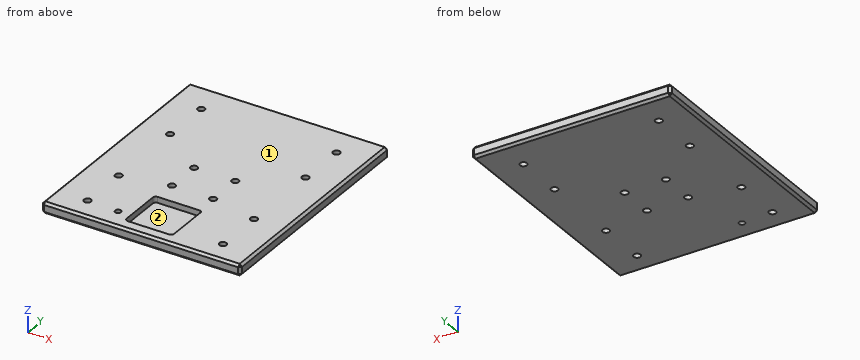
```python
from build123d import *

# Parameters (mm, degrees)
SKETCH1_W           = 107.95
SKETCH1_H           = 127
BOSS_EXTRUDE1_DEPTH = 6.223
CHAMFER1_SIZE       = 1.27
SKETCH2_R           = 1.905
CUT_EXTRUDE1_DEPTH  = 7.223
SKETCH3_R           = 1.905
CUT_EXTRUDE2_DEPTH  = 7.223
SKETCH4_W           = 25.781
SKETCH4_H           = 25.781
CUT_EXTRUDE3_DEPTH  = 3.175
FILLET1_R           = 1.5875
SKETCH5_R           = 1.5875
CUT_EXTRUDE4_DEPTH  = 7.223


with BuildPart() as part:
    # Sketch1 → Boss-Extrude1 (new body)
    with BuildSketch(Plane.XY):
        Rectangle(SKETCH1_W, SKETCH1_H)
    extrude(amount=BOSS_EXTRUDE1_DEPTH)

    # Chamfer1
    chamfer1_edges = [part.edges().sort_by_distance(p)[0] for p in [
        (-53.975, 0, 6.223),
        (0, -63.5, 6.223),
        (53.975, 0, 6.223),
        (0, -63.5, 0),
        (-53.975, 0, 0),
        (0, 63.5, 0),
        (53.975, 0, 0),
        (0, 63.5, 6.223),
        (53.975, -63.5, 3.1115),
        (-53.975, -63.5, 3.1115),
        (-53.975, 63.5, 3.1115),
        (53.975, 63.5, 3.1115),
    ]]
    chamfer(chamfer1_edges, length=CHAMFER1_SIZE)

    # Sketch2 → Cut-Extrude1 (cut, through all)
    with BuildSketch(Plane.XY.offset(6.223)):
        with Locations((-36.703, 46.228)):
            Circle(SKETCH2_R)
        with Locations((-36.703, -51.308)):
            Circle(SKETCH2_R)
        with Locations((36.703, -51.308)):
            Circle(SKETCH2_R)
        with Locations((36.703, 46.228)):
            Circle(SKETCH2_R)
        with Locations((-36.703, 19.558)):
            Circle(SKETCH2_R)
        with Locations((-36.703, -24.638)):
            Circle(SKETCH2_R)
        with Locations((36.703, 19.558)):
            Circle(SKETCH2_R)
        with Locations((36.703, -24.638)):
            Circle(SKETCH2_R)
    extrude(amount=-CUT_EXTRUDE1_DEPTH, mode=Mode.SUBTRACT)

    # Sketch3 → Cut-Extrude2 (cut, through all)
    with BuildSketch(Plane.XY.offset(6.223)):
        with Locations((-11.176, -0.254)):
            Circle(SKETCH3_R)
        with Locations((11.176, -0.254)):
            Circle(SKETCH3_R)
        with Locations((11.176, -19.304)):
            Circle(SKETCH3_R)
        with Locations((-11.176, -19.304)):
            Circle(SKETCH3_R)
    extrude(amount=-CUT_EXTRUDE2_DEPTH, mode=Mode.SUBTRACT)

    # Sketch4 → Cut-Extrude3 (cut)
    with BuildSketch(Plane.XY.offset(6.223)):
        with Locations((0, -44.2595)):
            Rectangle(SKETCH4_W, SKETCH4_H)
    extrude(amount=-CUT_EXTRUDE3_DEPTH, mode=Mode.SUBTRACT)

    # Fillet1
    fillet1_edges = [part.edges().sort_by_distance(p)[0] for p in [
        (12.8905, -31.369, 4.6355),
        (12.8905, -57.15, 4.6355),
        (-12.8905, -57.15, 4.6355),
        (-12.8905, -31.369, 4.6355),
    ]]
    fillet(fillet1_edges, radius=FILLET1_R)

    # Sketch5 → Cut-Extrude4 (cut, through all)
    with BuildSketch(Plane.XY.offset(6.223)):
        with Locations((-19.685, -52.07)):
            Circle(SKETCH5_R)
    extrude(amount=-CUT_EXTRUDE4_DEPTH, mode=Mode.SUBTRACT)


solid = part.part
```
For this review, take the finished solid that the model builds, in its own axes (mm). Face numbers are marked on the shaded views. Coordinates: 2 decimals unless noted, no trailing zeros. Put each result on its own line as item: value.
Q1. The part is to be moulded in two halves that separate along X. For the marked faces 1 and 2, say which applies: +X half, -X half, draft (parallel to the pull), parting line (faces both ways), or undercut.
From the geometry:
face 1: draft
face 2: undercut
Q2. Clearance check with a flat-ended pin moving along its axis: pin 1 Ø7.5 at (x, y) = (-2.5, -49) entering from +Z. State where the tip first meets the part, or that it passes through.
From the geometry:
pin 1: stops at z = 3.05
Q3. Wall thickness on L1, parallel to Y at x = -36.5, z = 4.75; L2, parallel to X at y = 46.5, z = 3 (3 decimals); L3, parallel to X at y = -55, z = 4.5 (1 decimal): over which ranges is each line inside the solid? List them lowest first.
From the geometry:
L1: y = -63.5 to -53.2, -49.41 to -26.53, -22.74 to 17.66, 21.45 to 44.33, 48.12 to 63.5
L2: x = -53.975 to -38.588, -34.818 to 34.818, 38.588 to 53.975
L3: x = -54 to -12.9, 12.9 to 54
